Geometry check sheet. Reference: the model listing, model coordinates, mm. A direction names the side the tool comes from. Round coordinates to 2 decimals unless told otherwise and drop trailing zeros. Use a Markdown table: item, result.
```python
from build123d import *

# Parameters (mm, degrees)
F0_R     = 1.6
F1_DEPTH = 6


with BuildPart() as f1:
    # F0 (on Right) → F1 (new body)
    with BuildSketch(Plane.YZ):
        with BuildLine():
            Line((0, 0.585502), (155, 0.585502))
            ThreePointArc((155, 0.585502), (158.535534, 2.049968), (160, 5.585502))
            Line((160, 5.585502), (160, 10.585502))
            Line((160, 10.585502), (166, 10.585502))
            Line((166, 10.585502), (166, 25.585502))
            Line((166, 25.585502), (160, 25.585502))
            Line((160, 25.585502), (160, 35.585502))
            Line((160, 35.585502), (166, 35.585502))
            Line((166, 35.585502), (166, 50.585502))
            Line((166, 50.585502), (160, 50.585502))
            Line((160, 50.585502), (160, 55.585502))
            ThreePointArc((160, 55.585502), (158.535534, 59.121036), (155, 60.585502))
            Line((155, 60.585502), (0, 60.585502))
            Line((0, 60.585502), (-155, 60.585502))
            ThreePointArc((-155, 60.585502), (-158.535534, 59.121036), (-160, 55.585502))
            Line((-160, 55.585502), (-160, 50.585502))
            Line((-160, 50.585502), (-166, 50.585502))
            Line((-166, 50.585502), (-166, 35.585502))
            Line((-166, 35.585502), (-160, 35.585502))
            Line((-160, 35.585502), (-160, 25.585502))
            Line((-160, 25.585502), (-166, 25.585502))
            Line((-166, 25.585502), (-166, 10.585502))
            Line((-166, 10.585502), (-160, 10.585502))
            Line((-160, 10.585502), (-160, 5.585502))
            ThreePointArc((-160, 5.585502), (-158.535534, 2.049968), (-155, 0.585502))
            Line((-155, 0.585502), (0, 0.585502))
        make_face()
        with Locations((-130, 10.585502)):
            Circle(F0_R, mode=Mode.SUBTRACT)
        with Locations((-120, 10.585502)):
            Circle(F0_R, mode=Mode.SUBTRACT)
        with Locations((-110, 10.585502)):
            Circle(F0_R, mode=Mode.SUBTRACT)
        with Locations((-100, 10.585502)):
            Circle(F0_R, mode=Mode.SUBTRACT)
        with Locations((-90, 10.585502)):
            Circle(F0_R, mode=Mode.SUBTRACT)
        with Locations((-80, 10.585502)):
            Circle(F0_R, mode=Mode.SUBTRACT)
        with Locations((-70, 10.585502)):
            Circle(F0_R, mode=Mode.SUBTRACT)
        with Locations((-60, 10.585502)):
            Circle(F0_R, mode=Mode.SUBTRACT)
        with Locations((-50, 10.585502)):
            Circle(F0_R, mode=Mode.SUBTRACT)
        with Locations((-40, 10.585502)):
            Circle(F0_R, mode=Mode.SUBTRACT)
        with Locations((-30, 10.585502)):
            Circle(F0_R, mode=Mode.SUBTRACT)
        with Locations((-20, 10.585502)):
            Circle(F0_R, mode=Mode.SUBTRACT)
        with Locations((-10, 10.585502)):
            Circle(F0_R, mode=Mode.SUBTRACT)
        with Locations((0, 10.585502)):
            Circle(F0_R, mode=Mode.SUBTRACT)
        with Locations((10, 10.585502)):
            Circle(F0_R, mode=Mode.SUBTRACT)
        with Locations((20, 10.585502)):
            Circle(F0_R, mode=Mode.SUBTRACT)
        with Locations((30, 10.585502)):
            Circle(F0_R, mode=Mode.SUBTRACT)
        with Locations((40, 10.585502)):
            Circle(F0_R, mode=Mode.SUBTRACT)
        with Locations((50, 10.585502)):
            Circle(F0_R, mode=Mode.SUBTRACT)
        with Locations((60, 10.585502)):
            Circle(F0_R, mode=Mode.SUBTRACT)
        with Locations((70, 10.585502)):
            Circle(F0_R, mode=Mode.SUBTRACT)
        with Locations((80, 10.585502)):
            Circle(F0_R, mode=Mode.SUBTRACT)
        with Locations((90, 10.585502)):
            Circle(F0_R, mode=Mode.SUBTRACT)
        with Locations((100, 10.585502)):
            Circle(F0_R, mode=Mode.SUBTRACT)
        with Locations((110, 10.585502)):
            Circle(F0_R, mode=Mode.SUBTRACT)
        with Locations((120, 10.585502)):
            Circle(F0_R, mode=Mode.SUBTRACT)
        with Locations((130, 10.585502)):
            Circle(F0_R, mode=Mode.SUBTRACT)
        with Locations((-140, 30.585502)):
            Circle(F0_R, mode=Mode.SUBTRACT)
        with Locations((-130, 30.585502)):
            Circle(F0_R, mode=Mode.SUBTRACT)
        with Locations((-120, 30.585502)):
            Circle(F0_R, mode=Mode.SUBTRACT)
        with Locations((-110, 30.585502)):
            Circle(F0_R, mode=Mode.SUBTRACT)
        with Locations((-100, 30.585502)):
            Circle(F0_R, mode=Mode.SUBTRACT)
        with Locations((-90, 30.585502)):
            Circle(F0_R, mode=Mode.SUBTRACT)
        with Locations((-80, 30.585502)):
            Circle(F0_R, mode=Mode.SUBTRACT)
        with Locations((-70, 30.585502)):
            Circle(F0_R, mode=Mode.SUBTRACT)
        with Locations((-60, 30.585502)):
            Circle(F0_R, mode=Mode.SUBTRACT)
        with Locations((-50, 30.585502)):
            Circle(F0_R, mode=Mode.SUBTRACT)
        with Locations((-40, 30.585502)):
            Circle(F0_R, mode=Mode.SUBTRACT)
        with Locations((-30, 30.585502)):
            Circle(F0_R, mode=Mode.SUBTRACT)
        with Locations((-20, 30.585502)):
            Circle(F0_R, mode=Mode.SUBTRACT)
        with Locations((-10, 30.585502)):
            Circle(F0_R, mode=Mode.SUBTRACT)
        with Locations((-130, 50.585502)):
            Circle(F0_R, mode=Mode.SUBTRACT)
        with Locations((-120, 50.585502)):
            Circle(F0_R, mode=Mode.SUBTRACT)
        with Locations((-110, 50.585502)):
            Circle(F0_R, mode=Mode.SUBTRACT)
        with Locations((-100, 50.585502)):
            Circle(F0_R, mode=Mode.SUBTRACT)
        with Locations((-90, 50.585502)):
            Circle(F0_R, mode=Mode.SUBTRACT)
        with Locations((-80, 50.585502)):
            Circle(F0_R, mode=Mode.SUBTRACT)
        with Locations((-70, 50.585502)):
            Circle(F0_R, mode=Mode.SUBTRACT)
        with Locations((-60, 50.585502)):
            Circle(F0_R, mode=Mode.SUBTRACT)
        with Locations((-50, 50.585502)):
            Circle(F0_R, mode=Mode.SUBTRACT)
        with Locations((-40, 50.585502)):
            Circle(F0_R, mode=Mode.SUBTRACT)
        with Locations((-30, 50.585502)):
            Circle(F0_R, mode=Mode.SUBTRACT)
        with Locations((-20, 50.585502)):
            Circle(F0_R, mode=Mode.SUBTRACT)
        with Locations((-10, 50.585502)):
            Circle(F0_R, mode=Mode.SUBTRACT)
        with Locations((0, 30.585502)):
            Circle(F0_R, mode=Mode.SUBTRACT)
        with Locations((10, 30.585502)):
            Circle(F0_R, mode=Mode.SUBTRACT)
        with Locations((20, 30.585502)):
            Circle(F0_R, mode=Mode.SUBTRACT)
        with Locations((30, 30.585502)):
            Circle(F0_R, mode=Mode.SUBTRACT)
        with Locations((40, 30.585502)):
            Circle(F0_R, mode=Mode.SUBTRACT)
        with Locations((50, 30.585502)):
            Circle(F0_R, mode=Mode.SUBTRACT)
        with Locations((60, 30.585502)):
            Circle(F0_R, mode=Mode.SUBTRACT)
        with Locations((70, 30.585502)):
            Circle(F0_R, mode=Mode.SUBTRACT)
        with Locations((80, 30.585502)):
            Circle(F0_R, mode=Mode.SUBTRACT)
        with Locations((90, 30.585502)):
            Circle(F0_R, mode=Mode.SUBTRACT)
        with Locations((100, 30.585502)):
            Circle(F0_R, mode=Mode.SUBTRACT)
        with Locations((110, 30.585502)):
            Circle(F0_R, mode=Mode.SUBTRACT)
        with Locations((120, 30.585502)):
            Circle(F0_R, mode=Mode.SUBTRACT)
        with Locations((130, 30.585502)):
            Circle(F0_R, mode=Mode.SUBTRACT)
        with Locations((140, 30.585502)):
            Circle(F0_R, mode=Mode.SUBTRACT)
        with Locations((0, 50.585502)):
            Circle(F0_R, mode=Mode.SUBTRACT)
        with Locations((10, 50.585502)):
            Circle(F0_R, mode=Mode.SUBTRACT)
        with Locations((20, 50.585502)):
            Circle(F0_R, mode=Mode.SUBTRACT)
        with Locations((30, 50.585502)):
            Circle(F0_R, mode=Mode.SUBTRACT)
        with Locations((40, 50.585502)):
            Circle(F0_R, mode=Mode.SUBTRACT)
        with Locations((50, 50.585502)):
            Circle(F0_R, mode=Mode.SUBTRACT)
        with Locations((60, 50.585502)):
            Circle(F0_R, mode=Mode.SUBTRACT)
        with Locations((70, 50.585502)):
            Circle(F0_R, mode=Mode.SUBTRACT)
        with Locations((80, 50.585502)):
            Circle(F0_R, mode=Mode.SUBTRACT)
        with Locations((90, 50.585502)):
            Circle(F0_R, mode=Mode.SUBTRACT)
        with Locations((100, 50.585502)):
            Circle(F0_R, mode=Mode.SUBTRACT)
        with Locations((110, 50.585502)):
            Circle(F0_R, mode=Mode.SUBTRACT)
        with Locations((120, 50.585502)):
            Circle(F0_R, mode=Mode.SUBTRACT)
        with Locations((130, 50.585502)):
            Circle(F0_R, mode=Mode.SUBTRACT)
    extrude(amount=F1_DEPTH)


solid = f1.part
```
Item 1: Material ranges on line 1 along Z through (x, y) = (3.1, 70); line 2 along Z through (x, y) = (3.9, -1); line 3 along Y through (x, z) = (4.75, 6.5), recorded low to high. Write a range as from..to.
Outcome:
| item | result |
|---|---|
| line 1 | z = 0.59..8.99, 12.19..28.99, 32.19..48.99, 52.19..60.59 |
| line 2 | z = 0.59..9.34, 11.83..29.34, 31.83..49.34, 51.83..60.59 |
| line 3 | y = -160..160 |
Item 2: Cross-section at A-A, the plane x = 4.5. Count the separate pieces of the cut face and the enclosed holes in it, and give its area (3 significant figures).
Outcome:
| item | result |
|---|---|
| separate pieces | 1 |
| enclosed holes | 83 |
| area | 18,900 mm2 |
Item 3: Go/stop test with flat-tipped pins: pin 1 (5 mm diameter, centred on y = -70, z = 10.59, fed in from -X); pin 2 (1.8 mm diameter, centred on x = 3, y = 162.5, fed in from +Z). Record where each tip stops, or that it passes through.
Outcome:
| item | result |
|---|---|
| pin 1 | stops at x = 0 |
| pin 2 | stops at z = 50.59 |
Item 4: Access from +Z, -Z, +X, -X, +Y, -Y to the whole of each face (thin tool, end or side, straight path). Record for faces 1 (the face through (3, -163, 10.586)), 2 (the face through (3, 163, 35.586)), 3 (the face through (3, 163, 50.586)).
Outcome:
| item | result |
|---|---|
| face 1 | -Z, +X, -X, -Y |
| face 2 | +X, -X, +Y |
| face 3 | +Z, +X, -X, +Y |
Item 5: Mould release check, pull along Z, two halves, no side actions. Record for faces 4 (the face through (3, 163, 10.586)), 5 (the face through (3, -163, 50.586)), 6 (the face through (3, 160, 31)): +Z half, -Z half, draft (parallel to the pull), parting line (faces both ways), or undercut.
Outcome:
| item | result |
|---|---|
| face 4 | -Z half |
| face 5 | +Z half |
| face 6 | undercut |
